Autodesk Inventor part; units mm, degrees
ref_plane "YZ Plane" through (0, 0, 0) normal (1, 0, 0) x (0, 1, 0)
ref_plane "XZ Plane" through (0, 0, 0) normal (0, 1, 0) x (-1, 0, 0)
ref_plane "XY Plane" through (0, 0, 0) normal (0, 0, 1) x (1, 0, 0)
sketch "Skizze1" plane through (0, 0, 0) normal (0, 0, 1) x (1, 0, 0)
  line L0 (112, -64) -> (-112, -64)
  line L1 (-114, -66) -> (114, -66)
  line L2 (114, -64) -> (-114, 64) construction
  line L3 (114, 64) -> (-114, -64) construction
  line L4 (115, -70) -> (-115, -70)
  line L5 (-116, 66) -> (116, -66) construction
  line L6 (-116, -66) -> (116, 66) construction
  line L7 (120, -70) -> (-120, 70) construction
  line L8 (120, 70) -> (-120, -70) construction
  line L9 (-112, 64) -> (112, 64)
  line L10 (-115, 70) -> (115, 70)
  line L11 (114, 66) -> (-114, 66)
  line L12 (-116, 64) -> (-116, -64)
  arc A0 (-116, -64) -> (-114, -66) centre (-114, -64) ccw
  line L13 (-114, -62) -> (-114, 62)
  arc A1 (-114, -62) -> (-112, -64) centre (-112, -62) ccw
  arc A2 (-120, -65) -> (-115, -70) centre (-115, -65) ccw
  line L14 (-120, -65) -> (-120, 65)
  arc A3 (-115, 70) -> (-120, 65) centre (-115, 65) ccw
  arc A4 (-114, 66) -> (-116, 64) centre (-114, 64) ccw
  arc A5 (-112, 64) -> (-114, 62) centre (-112, 62) ccw
  arc A6 (120, 65) -> (115, 70) centre (115, 65) ccw
  line L15 (120, 65) -> (120, -65)
  arc A7 (115, -70) -> (120, -65) centre (115, -65) ccw
  arc A8 (112, -64) -> (114, -62) centre (112, -62) ccw
  arc A9 (114, 62) -> (112, 64) centre (112, 62) ccw
  line L16 (114, 62) -> (114, -62)
  arc A10 (114, -66) -> (116, -64) centre (114, -64) ccw
  arc A11 (116, 64) -> (114, 66) centre (114, 64) ccw
  line L17 (116, -64) -> (116, 64)
  line L18 (-160, -110) -> (160, -110)
  line L19 (160, -110) -> (160, 110)
  line L20 (160, 110) -> (-160, 110)
  line L21 (-160, 110) -> (-160, -110)
  line L22 (-160, -110) -> (160, 110) construction
  line L23 (160, -110) -> (-160, 110) construction
  circle A12 centre (-140, -90) radius 3.25
  line L24 (140, 90) -> (-140, 90)
  line L25 (-140, 90) -> (-140, -90)
  line L26 (-140, -90) -> (140, -90)
  line L27 (140, -90) -> (140, 90)
  line L28 (140, 90) -> (-140, -90) construction
  line L29 (-140, 90) -> (140, -90) construction
  circle A13 centre (140, -90) radius 3.25
  circle A14 centre (140, 90) radius 3.25
  circle A15 centre (-140, 90) radius 3.25
  point P0 (0, 0)
  point P1 (0, 0)
  point P2 (0, 0)
  point P3 (0, 0)
  point P4 (0, 0)
  point P5 (0, 0)
  point P6 (0, 0)
  point P7 (0, 0)
  point P8 (0, 0)
  dimension "d0" = 140
  dimension "d1" = 240
  dimension "d2" = 5
  dimension "d3" = 232
  dimension "d4" = 132
  dimension "d5" = 2
  dimension "d6" = 128
  dimension "d7" = 228
  dimension "d8" = 2
  dimension "d9" = 40
  dimension "d10" = 40
  dimension "d11" = 6.5
  dimension "d12" = 20
  dimension "d13" = 20
extrude "Extrusion1" add sketch "Skizze1" along normal blind 6 contours A0 L12 A4 L11 A11 L17 A10 L1 | L4 A2 L14 A3 L10 A6 L15 A7 | L21 L20 L19 L18 | L26 L25 A12 | A12 L25 L26 | A12 L25 A15 L24 A14 L27 A13 L26 | A13 L27 L26 | L26 L27 A13 | A15 L24 L25 | L25 L24 A15 | A14 L24 L27 | L27 L24 A14
extrude "Extrusion2" cut sketch "Skizze1" along normal through all contours L26 L25 A12 | A12 L25 L26 | A13 L27 L26 | L26 L27 A13 | A15 L24 L25 | L25 L24 A15 | A14 L24 L27 | L27 L24 A14
equation "\"d14\" = mdf_thickness"
equation "\"d16\" = mdf_thickness"
equation "\"kg_thickness\" = 4.9"
equation "\"ht_thickness\" = 1.9"
equation "\"case_thickness\" = 18"
equation "\"inner_thickness\" = 15"
equation "\"gap_fit\" = 0.1"
equation "\"gap_slide\" = 0.2"
equation "\"gap_air\" = 1"
equation "\"bore_diameter\" = 73"
equation "\"mdf_thickness\" = 6"
equation "\"tape_width\" = 15"
equation "\"tape_thickness\" = 3"
equation "\"inner_depth\" = 255"
properties part number "Flachfaltenfilter_Basis"
For this review, take the finished solid that the model builds, in its own axes (mm). A direction names the side the tool comes from. Give positions to 0.01 mm unless a question says otherwise; leave off trailing zeros. Order: outer loops, then holes, each group sorted by start corner. A loop starts at its lowest first (then second) coordinate and runs counter-clockwise, first axis right, second up.
1) For faces 1 (the face through (2, -64, 3)), 2 (the face through (-2, 75, 6)), list the 3-axis set-ups (+Z, -Z, +X, -X, +Y, -Y) from which the entire face can be reached by the end or side of a thin tool; tool diameter is ignored.
2) Take a section at C-C (y = 90). Give the boundary of the cut face in (x, z), then the cut area to 3 significant figures.
3) Insertion check: pin 1 (4 mm diameter, centred on x = 140, y = -90, fed in from -Z). The pin has a flat end and moves straight along its axis. Give the tip position at first contact, or say it passes through.
4) Take a section at D-D (x = -140). Give the boundary of the cut face in (y, z).
5) Take a section at A-A (x = -49). Give the boundary of the cut face in (y, z).
6) The part is to be moulded in two halves that separate along Y. For faces 3 (the face through (-2, -110, 3)), 4 (the face through (160, -2, 3)), 5 (the face through (114, 1, 3)), 6 (the face through (141.5, -87.117, 2.958)), say which applies: released by +Y, released by -Y, zero draft, split by the parting line, or undercut.
7) Take a section at B-B (z = 4.2). Give the boundary of the cut face in (x, y).
8) Wall thickness on line 1 (Y direction, x = 140, z = 3.85); line 2 (X direction, y = -90, z = 4.6); line 3 (Y direction, x = 8, z = 1): over which ranges is each line inside the solid? List them lowest first.
Derived:
1. face 1: +Z, -Z
1. face 2: +Z, +X, -X, +Y, -Y
2. outline: (-160, 0) - (-143.25, 0) - (-143.25, 6) - (-160, 6) - close; (-136.75, 0) - (136.75, 0) - (136.75, 6) - (-136.75, 6) - close; (143.25, 0) - (160, 0) - (160, 6) - (143.25, 6) - close
2. area: 1,840 mm2
3. pin 1: passes through
4. outline: (-110, 0) - (-93.25, 0) - (-93.25, 6) - (-110, 6) - close; (-86.75, 0) - (86.75, 0) - (86.75, 6) - (-86.75, 6) - close; (93.25, 0) - (110, 0) - (110, 6) - (93.25, 6) - close
5. outline: (-110, 0) - (-64, 0) - (-64, 6) - (-110, 6) - close; (64, 0) - (110, 0) - (110, 6) - (64, 6) - close
6. face 3: released by -Y
6. face 4: zero draft
6. face 5: undercut
6. face 6: undercut
7. outline: (-160, -110) - (160, -110) - (160, 110) - (-160, 110) - close; hole circle Ø6.5 at (-140, -90); hole circle Ø6.5 at (-140, 90); hole (-114, -62) arc R2 ccw to (-112, -64) - (112, -64) arc R2 ccw to (114, -62) - (114, 62) arc R2 ccw to (112, 64) - (-112, 64) arc R2 ccw to (-114, 62) - close; hole circle Ø6.5 at (140, -90); hole circle Ø6.5 at (140, 90)
8. line 1: y = -110 to -93.25, -86.75 to 86.75, 93.25 to 110
8. line 2: x = -160 to -143.25, -136.75 to 136.75, 143.25 to 160
8. line 3: y = -110 to -64, 64 to 110
